Part model, mm, in its own coordinate system. Face numbers are marked on the shaded views. A direction names the side the tool comes from. Round coordinates to 2 decimals unless told otherwise and drop trailing zeros. Loops run counter-clockwise (first coordinate to the right, second up) from the corner with the lowest first, then second, coordinate; pieces in that order, holes last.
1) Mould opens along Z. For the marked faces 6, 7 and 8 say: +Z half, -Z half, draft (parallel to the pull), parting line (faces both ways), or undercut.
2) 3-axis set-ups, long thin cutter, end or side, ignore diameter. For the marked faces 1, 2, 3, 4 and 5: which of +Z, -Z, +X, -X, +Y, -Y reach the whole face in a straight line?
3) Drop flat-ended pins along their axis: P1, Ø3.5, axis at x = 9, z = 5.5, coming from the -Y side; P2, Ø3.5, axis at x = 12.5, y = 3, coming from the -Z side; P3, Ø4, axis at x = 10, z = 6, coming from the +Y side; P4, Ø1, axis at x = 3.5, y = 35.5, coming from the -Z side. Give the stop position or say it passes through.
4) Band-saw the part on D-D, the plane z = 8.5. Write the cut outline in (x, y).
5) Probe line 1 (Y direction, x = 3.5, z = 4.5); line 2 (Y direction, x = 8, z = 8.25); line 3 (Y direction, x = 11.5, z = 8.7). List the from-to ranges inside material, lowest first.
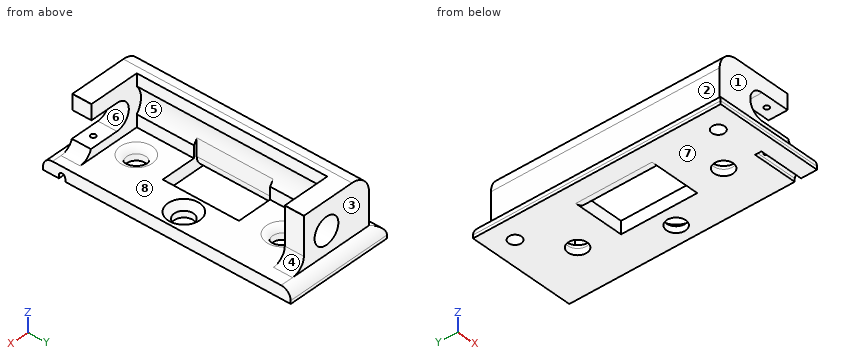
from build123d import *

# Parameters (mm, degrees)
ESQUISSE1_W                  = 17
ESQUISSE1_H                  = 39
BOSS_EXTRU_1_DEPTH           = 2
ESQUISSE2_W                  = 8
ESQUISSE2_H                  = 3
ESQUISSE2_W_2                = 9
BOSS_EXTRU_2_DEPTH           = 8
ESQUISSE3_R                  = 2.1
ENL_V_MAT_EXTRU_1_DEPTH      = 43.367037979
CONG_1_R                     = 0.0326
ESQUISSE14_W                 = 4
ESQUISSE14_H                 = 35.996211904
BOSS_EXTRU_8_DEPTH           = 8
ENL_V_MAT_EXTRU_2_DEPTH      = 3
ENL_V_MAT_EXTRU_2_DEPTH_BACK = 44.289721644
ESQUISSE4_W                  = 6
ESQUISSE4_H                  = 12
ENL_V_START                  = -3
ESQUISSE15_R                 = 3.25
ENL_V_MAT_EXTRU_7_DEPTH      = 29.95
CONG_9_R                     = 3
CONG_10_R                    = 2
CONG_11_R                    = 2
CONG_12_R                    = 1.5
ESQUISSE16_R                 = 1
ENL_V_MAT_EXTRU_8_DEPTH      = 8
ENL_V_MAT_EXTRU_9_REACH      = 44.367
ESQUISSE17_W                 = 6.298788147
ESQUISSE17_H                 = 4.2
ENL_V_START_2                = -0.5
ESQUISSE18_R                 = 0.4
ENL_V_MAT_EXTRU_10_DEPTH     = 10
ENL_V_MAT_EXTRU_18_DEPTH     = 7
ESQUISSE21_R                 = 1.5
ENL_V_MAT_EXTRU_19_DEPTH     = 44.289721683
CHANFREIN1_SIZE              = 1
ENL_V_MAT_EXTRU_20_REACH     = 45.29
ESQUISSE22_R                 = 1.5
CONG_14_R                    = 1


with BuildPart() as part:
    # Esquisse1 → Boss.-Extru.1 (new body)
    with BuildSketch(Plane.XY):
        with Locations((8.5, 19.5)):
            Rectangle(ESQUISSE1_W, ESQUISSE1_H)
    extrude(amount=BOSS_EXTRU_1_DEPTH)

    # Esquisse2 → Boss.-Extru.2 (add)
    with BuildSketch(Plane.XY.offset(2)):
        with Locations((9, 36)):
            Rectangle(ESQUISSE2_W, ESQUISSE2_H)
        with Locations((9, 3.003788096)):
            Rectangle(ESQUISSE2_W_2, ESQUISSE2_H)
    extrude(amount=BOSS_EXTRU_2_DEPTH)

    # Esquisse3 → Enlèv. mat.-Extru.1 (cut, through all)
    with BuildSketch(Plane.XZ.offset(-1.503788096)):
        with Locations(Location((9, 5.5, 0), (0, 0, 270))):
            Circle(ESQUISSE3_R)
    extrude(amount=-ENL_V_MAT_EXTRU_1_DEPTH, mode=Mode.SUBTRACT)

    # Congé1
    cong_1_edges = [part.edges().sort_by_distance(p)[0] for p in [
        (13, 36, 10),
        (13.5, 3.003788096, 10),
    ]]
    fillet(cong_1_edges, radius=CONG_1_R)

    # Esquisse14 → Boss.-Extru.8 (add)
    with BuildSketch(Plane.XY.offset(2)):
        with Locations((3.5, 19.501894048)):
            Rectangle(ESQUISSE14_W, ESQUISSE14_H)
    extrude(amount=BOSS_EXTRU_8_DEPTH)

    # Esquisse4 → Enlèv. mat.-Extru.2 (cut, two sides: drawn at the far end of the back side and taken through both)
    with BuildSketch(Plane.XY.offset(2).offset(-ENL_V_MAT_EXTRU_2_DEPTH_BACK)):
        with Locations((8, 19.5)):
            Rectangle(ESQUISSE4_W, ESQUISSE4_H)
    extrude(amount=ENL_V_MAT_EXTRU_2_DEPTH + ENL_V_MAT_EXTRU_2_DEPTH_BACK, mode=Mode.SUBTRACT)

    # Esquisse15 → Enlèv. mat.-Extru.7 (cut)
    with BuildSketch(Plane.XZ.offset(-1.503788096).offset(ENL_V_START)):
        with Locations((8, 6)):
            Circle(ESQUISSE15_R)
    extrude(amount=-ENL_V_MAT_EXTRU_7_DEPTH, mode=Mode.SUBTRACT)

    # Congé9
    cong_9_edges = [part.edges().sort_by_distance(p)[0] for p in [
        (1.5, 19.501894048, 10),
    ]]
    fillet(cong_9_edges, radius=CONG_9_R)

    # Congé10
    cong_10_edges = [part.edges().sort_by_distance(p)[0] for p in [
        (5, 19.5, 0),
    ]]
    fillet(cong_10_edges, radius=CONG_10_R)

    # Congé11
    cong_11_edges = [part.edges().sort_by_distance(p)[0] for p in [
        (13, 36, 2),
        (13.5, 3.003788096, 2),
    ]]
    fillet(cong_11_edges, radius=CONG_11_R)

    # Congé12
    cong_12_edges = [part.edges().sort_by_distance(p)[0] for p in [
        (8.5, 39, 2),
        (0, 19.5, 2),
        (8.5, 0, 2),
    ]]
    fillet(cong_12_edges, radius=CONG_12_R - 0.0001)  # a hair under: the kernel refuses the full size

    # Esquisse16 → Enlèv. mat.-Extru.8 (cut)
    with BuildSketch(Plane(origin=(0, 0, 0), x_dir=(-1, 0, 0), z_dir=(0, 0, -1))):
        with Locations((-3.5, 35.5)):
            Circle(ESQUISSE16_R)
        with Locations((-3.5, 3.5)):
            Circle(ESQUISSE16_R)
    extrude(amount=-ENL_V_MAT_EXTRU_8_DEPTH, mode=Mode.SUBTRACT)

    # Esquisse17 → Enlèv. mat.-Extru.9 (cut, up to next)
    with BuildSketch(Plane.XZ.offset(-1.503788096), mode=Mode.PRIVATE) as enl_v_mat_extru_9_sk1:
        with Locations((12.149394074, 5.5)):
            Rectangle(ESQUISSE17_W, ESQUISSE17_H)
    enl_v_mat_extru_9_tool1 = extrude(enl_v_mat_extru_9_sk1.sketch, amount=-ENL_V_MAT_EXTRU_9_REACH, mode=Mode.PRIVATE) & part.part
    add(enl_v_mat_extru_9_tool1.solids().sort_by_distance((12.149394, 1.503788, 5.5))[0], mode=Mode.SUBTRACT)

    # Esquisse18 → Enlèv. mat.-Extru.10 (cut)
    with BuildSketch(Plane.XY.offset(10).offset(ENL_V_START_2)):
        with Locations((11.5, 3.003788096)):
            Circle(ESQUISSE18_R)
    extrude(amount=-ENL_V_MAT_EXTRU_10_DEPTH, mode=Mode.SUBTRACT)

    # Esquisse20 → Enlèv. mat.-Extru.18 (cut)
    with BuildSketch(Plane(origin=(17, 0, 0), x_dir=(0, 0, -1), z_dir=(1, 0, 0))):
        with BuildLine():
            Line((-0.5, 3.503788096), (1.040895872, 3.503788096))
            ThreePointArc((1.040895872, 3.503788096), (1.540895872, 3.003788096), (1.040895872, 2.503788096))
            Line((1.040895872, 2.503788096), (-0.5, 2.503788096))
            ThreePointArc((-0.5, 2.503788096), (-1, 3.003788096), (-0.5, 3.503788096))
        make_face()
    extrude(amount=-ENL_V_MAT_EXTRU_18_DEPTH, mode=Mode.SUBTRACT)

    # Esquisse21 → Enlèv. mat.-Extru.19 (cut, through all)
    with BuildSketch(Plane.XY.offset(2)):
        with Locations((14, 19.5)):
            Circle(ESQUISSE21_R)
    extrude(amount=-ENL_V_MAT_EXTRU_19_DEPTH, mode=Mode.SUBTRACT)

    # Chanfrein1
    chanfrein1_edges = [part.edges().sort_by_distance(p)[0] for p in [
        (12.5, 19.5, 2),
    ]]
    chamfer(chanfrein1_edges, length=CHANFREIN1_SIZE)

    # Esquisse22 → Enlèv. mat.-Extru.20 (cut, up to next)
    with BuildSketch(Plane.XY.offset(2), mode=Mode.PRIVATE) as enl_v_mat_extru_20_sk1:
        with Locations((9.5, 31)):
            Circle(ESQUISSE22_R)
    enl_v_mat_extru_20_tool1 = extrude(enl_v_mat_extru_20_sk1.sketch, amount=-ENL_V_MAT_EXTRU_20_REACH, mode=Mode.PRIVATE) & part.part
    # Esquisse22 → Enlèv. mat.-Extru.20 (cut, up to next)
    with BuildSketch(Plane.XY.offset(2), mode=Mode.PRIVATE) as enl_v_mat_extru_20_sk2:
        with Locations((9.5, 8.003788096)):
            Circle(ESQUISSE22_R)
    enl_v_mat_extru_20_tool2 = extrude(enl_v_mat_extru_20_sk2.sketch, amount=-ENL_V_MAT_EXTRU_20_REACH, mode=Mode.PRIVATE) & part.part
    add(enl_v_mat_extru_20_tool1.solids().sort_by_distance((9.5, 31, 2))[0], mode=Mode.SUBTRACT)
    add(enl_v_mat_extru_20_tool2.solids().sort_by_distance((9.5, 8.003788, 2))[0], mode=Mode.SUBTRACT)

    # Congé14
    cong_14_edges = [part.edges().sort_by_distance(p)[0] for p in [
        (8, 31, 2),
        (8, 8.003788096, 2),
    ]]
    fillet(cong_14_edges, radius=CONG_14_R)


solid = part.part
Reported:
1. face 6: undercut
1. face 7: -Z half
1. face 8: +Z half
2. face 1: +Z, +X, -X, -Y
2. face 2: +Z, -X, +Y, -Y
2. face 3: +Z, +X, -X, +Y
2. face 4: +Z, +X, +Y
2. face 5: +X
3. P1: passes through
3. P2: stops at z = 0
3. P3: stops at y = 37.5
3. P4: stops at z = 8
4. outline: (1.9, 1.5) - (13.5, 1.5) - (13.5, 4.5) - (5.5, 4.5) - (5.5, 34.5) - (13, 34.5) - (13, 37.5) - (1.9, 37.5) - close; hole circle Ø0.8 at (11.5, 3)
5. line 1: y = 1.5 to 2.5, 4.5 to 34.5, 36.5 to 37.5
5. line 2: y = 1.5 to 4.5, 34.5 to 37.5
5. line 3: y = 1.5 to 2.6, 3.4 to 4.5, 34.5 to 37.5
